from build123d import *

# Parameters (mm, degrees)
CYLINDER003_R     = 18
CYLINDER003_DEPTH = 80
CYLINDER002_R     = 18
CYLINDER002_DEPTH = 80
CYLINDER005_R     = 18
CYLINDER005_DEPTH = 80
CYLINDER004_R     = 18
CYLINDER004_DEPTH = 80
CYLINDER001_R     = 18
CYLINDER001_DEPTH = 80
CYLINDER_R        = 18
CYLINDER_DEPTH    = 80
BOX_W             = 230
BOX_H             = 110
BOX_DEPTH         = 76


with BuildPart() as cylinder003:
    # Cylinder003 → Cylinder003 (new body)
    with BuildSketch(Plane(origin=(43, 79, 0), x_dir=(1, 0, 0), z_dir=(0, 0, 1))):
        Circle(CYLINDER003_R)
    extrude(amount=CYLINDER003_DEPTH)


with BuildPart() as fusion001:
    # Cylinder002 → Cylinder002 (new body)
    with BuildSketch(Plane(origin=(43, 31, 0), x_dir=(1, 0, 0), z_dir=(0, 0, 1))):
        Circle(CYLINDER002_R)
    extrude(amount=CYLINDER002_DEPTH)

    # Fusion001: union Cylinder003
    add(cylinder003.part)


with BuildPart() as fusion001_1:
    # Fusion001 placement: moved
    add(fusion001.part.moved(Location((72, 0, 0))))


with BuildPart() as cylinder005:
    # Cylinder005 → Cylinder005 (new body)
    with BuildSketch(Plane(origin=(43, 79, 0), x_dir=(1, 0, 0), z_dir=(0, 0, 1))):
        Circle(CYLINDER005_R)
    extrude(amount=CYLINDER005_DEPTH)


with BuildPart() as fusion002:
    # Cylinder004 → Cylinder004 (new body)
    with BuildSketch(Plane(origin=(43, 31, 0), x_dir=(1, 0, 0), z_dir=(0, 0, 1))):
        Circle(CYLINDER004_R)
    extrude(amount=CYLINDER004_DEPTH)

    # Fusion002: union Cylinder005
    add(cylinder005.part)


with BuildPart() as fusion002_1:
    # Fusion002 placement: moved
    add(fusion002.part.moved(Location((144, 0, 0))))


with BuildPart() as cylinder001:
    # Cylinder001 → Cylinder001 (new body)
    with BuildSketch(Plane(origin=(43, 79, 0), x_dir=(1, 0, 0), z_dir=(0, 0, 1))):
        Circle(CYLINDER001_R)
    extrude(amount=CYLINDER001_DEPTH)


with BuildPart() as fusion003:
    # Cylinder → Cylinder (new body)
    with BuildSketch(Plane(origin=(43, 31, 0), x_dir=(1, 0, 0), z_dir=(0, 0, 1))):
        Circle(CYLINDER_R)
    extrude(amount=CYLINDER_DEPTH)

    # Fusion: union Cylinder001
    add(cylinder001.part)

    # Fusion003: union Fusion001, Fusion002
    add(fusion001_1.part)
    add(fusion002_1.part)


with BuildPart() as fusion003_1:
    # Fusion003 placement: moved
    add(fusion003.part.moved(Location((0, 0, 10))))


with BuildPart() as cut:
    # Box → Box (new body)
    with BuildSketch(Plane.XY):
        with Locations((115, 55)):
            Rectangle(BOX_W, BOX_H)
    extrude(amount=BOX_DEPTH)

    # Cut: cut Fusion003
    add(fusion003_1.part, mode=Mode.SUBTRACT)


solid = cut.part
Read the model definition and answer for the solid it produces. Units are mm, in the model's axes. A direction names the side the tool comes from. Round coordinates to 2 decimals unless told otherwise and drop trailing zeros. Write each loop counter-clockwise with the first axis right and the second up, starting at its lowest first coordinate (ties: lowest second). Pieces come first, ordered by that corner, then holes. Notation, with made-up numbers: (52, 48) - (57, 48) arc R28 ccw to (57, 68) - close; hole circle Ø2 at (64.25, 33.5). An arc over 180 degrees is marked (long way). Use a Markdown table: item, result.
(1) Straight lines are drawn through the part: line 1 along X through (y, z) = (79, 51); line 2 along Y through (x, z) = (187, 27); line 3 along X through (y, z) = (81, 46). For each, find the intervals that lie inside material, in ascending order. Write a range as [from, to].
Reported:
| item | result |
|---|---|
| line 1 | [0, 25], [61, 97], [133, 169], [205, 230] |
| line 2 | [0, 13], [49, 61], [97, 110] |
| line 3 | [0, 25.11], [60.89, 97.11], [132.89, 169.11], [204.89, 230] |
(2) Which of the six approach directions +Z, -Z, +X, -X, +Y, -Y give full straight-line access (tool end or side, diameter ignored) to faces 1 (the flat face through (0, 54, 37)), 2 (the flat face through (43, 79, 10))?
Reported:
| item | result |
|---|---|
| face 1 | +Z, -Z, -X, +Y, -Y |
| face 2 | +Z |
(3) The mould has two halves that part along X. Classify faces 3 (the cylindrical face through (204.169, 84.407, 42.538)), 4 (the cylindrical face through (131.63, 24.11, 42.54)), 5 (the flat face through (113, 56, 76)), 6 (the flat face through (230, 54, 37)): released by +X, released by -X, zero draft, split by the parting line, or undercut.
Reported:
| item | result |
|---|---|
| face 3 | undercut |
| face 4 | undercut |
| face 5 | zero draft |
| face 6 | released by +X |
(4) The part is cut by section A-A (z = 25). Write down the section's boundary in (x, y).
Reported:
| item | result |
|---|---|
| outline | (0, 0) - (230, 0) - (230, 110) - (0, 110) - close; hole circle Ø36 at (43, 31); hole circle Ø36 at (43, 79); hole circle Ø36 at (115, 31); hole circle Ø36 at (115, 79); hole circle Ø36 at (187, 31); hole circle Ø36 at (187, 79) |
(5) The part is cut by section C-C (y = 31). Write down the section's boundary in (x, z).
Reported:
| item | result |
|---|---|
| outline | (0, 0) - (230, 0) - (230, 76) - (205, 76) - (205, 10) - (169, 10) - (169, 76) - (133, 76) - (133, 10) - (97, 10) - (97, 76) - (61, 76) - (61, 10) - (25, 10) - (25, 76) - (0, 76) - close |
(6) This flat-tipped pin is pushed along its axis until it touches: pin 1 Ø18 at (x, y) = (39, 84.5) entering from +Z. Where does it stop, or does it pass through?
Reported:
| item | result |
|---|---|
| pin 1 | z = 10 |
(7) The part is cut by section D-D (x = 49). Write down the section's boundary in (y, z).
Reported:
| item | result |
|---|---|
| outline | (0, 0) - (110, 0) - (110, 76) - (95.97, 76) - (95.97, 10) - (62.03, 10) - (62.03, 76) - (47.97, 76) - (47.97, 10) - (14.03, 10) - (14.03, 76) - (0, 76) - close |
(8) The part is cut by section B-B (x = 115). Write down the section's boundary in (y, z), then the cut area to 3 significant figures.
Reported:
| item | result |
|---|---|
| outline | (0, 0) - (110, 0) - (110, 76) - (97, 76) - (97, 10) - (61, 10) - (61, 76) - (49, 76) - (49, 10) - (13, 10) - (13, 76) - (0, 76) - close |
| area | 3,610 mm2 |
